```python
from build123d import *

# Parameters (mm, degrees)
BOSS_EXTRUDE1_DEPTH = 0.8
SKETCH2_W           = 9.888461937
SKETCH2_H           = 20
CUT_EXTRUDE1_DEPTH  = 0.8
FILLET1_R           = 1
BOSS_EXTRUDE2_DEPTH = 1
SKETCH4_W           = 5
SKETCH4_H           = 1
BOSS_EXTRUDE3_DEPTH = 1
FILLET2_R           = 1
CUT_EXTRUDE2_DEPTH  = 10


with BuildPart() as part:
    # Sketch1 → Boss-Extrude1 (new body)
    with BuildSketch(Plane(origin=(0, 0, 0), x_dir=(1, 0, 0), z_dir=(0, 1, 0))):
        Polygon((-22, 15), (-23.5, 4.326945416), (-23.5, -4.326945416), (-22, -15), (22, -15), (23.5, -4.326945416), (23.5, 4.326945416), (22, 15), align=None)
    extrude(amount=BOSS_EXTRUDE1_DEPTH)

    # Sketch2 → Cut-Extrude1 (cut)
    with BuildSketch(Plane(origin=(0, 0.8, 0), x_dir=(1, 0, 0), z_dir=(0, 1, 0))):
        with Locations((-21.444230969, 2.5)):
            Rectangle(SKETCH2_W, SKETCH2_H)
    extrude(amount=-CUT_EXTRUDE1_DEPTH, mode=Mode.SUBTRACT)

    # Fillet1
    fillet1_edges = [part.edges().sort_by_distance(p)[0] for p in [
        (-16.5, 0.4, 7.5),
    ]]
    fillet(fillet1_edges, radius=FILLET1_R)

    # Sketch3 → Boss-Extrude2 (add)
    with BuildSketch(Plane.XZ):
        Polygon((-19.5, 13.5), (-20.5, 13.5), (-20.5, 12.5), (-20.5, 8.5), (-19.5, 8.5), (-19.5, 12.5), (-15.5, 12.5), (-15.5, 13.5), align=None)
        Polygon((19.5, 13.5), (15.5, 13.5), (15.5, 12.5), (19.5, 12.5), (19.5, 8.5), (20.5, 8.5), (20.5, 12.5), (20.5, 13.5), align=None)
        Polygon((19.5, -13.5), (20.5, -13.5), (20.5, -12.5), (20.5, -8.5), (19.5, -8.5), (19.5, -12.5), (15.5, -12.5), (15.5, -13.5), align=None)
    extrude(amount=BOSS_EXTRUDE2_DEPTH)

    # Sketch4 → Boss-Extrude3 (add)
    with BuildSketch(Plane.XZ):
        with Locations((-18, -13)):
            Rectangle(SKETCH4_W, SKETCH4_H)
    extrude(amount=BOSS_EXTRUDE3_DEPTH)

    # Fillet2
    fillet2_edges = [part.edges().sort_by_distance(p)[0] for p in [
        (-16.5, 0.4, -12.5),
    ]]
    fillet(fillet2_edges, radius=FILLET2_R)

    # Sketch5 → Cut-Extrude2 (cut)
    with BuildSketch(Plane(origin=(0, 0.8, 0), x_dir=(1, 0, 0), z_dir=(0, 1, 0))):
        Polygon((1.1702653, 5.066019343), (0.081403121, 5.066019343), (2.306192784, 9.380762933), (3.209337816, 9.380762933), (5.432855444, 5.066019343), (4.3452653, 5.066019343), (2.7577653, 8.145616699), align=None)
        Polygon((1.1702653, -6.924365272), (0.081403121, -6.924365272), (2.306192784, -2.609621682), (3.209337816, -2.609621682), (5.432855444, -6.924365272), (4.3452653, -6.924365272), (2.7577653, -3.844767916), align=None)
    extrude(amount=-CUT_EXTRUDE2_DEPTH, mode=Mode.SUBTRACT)


solid = part.part
```
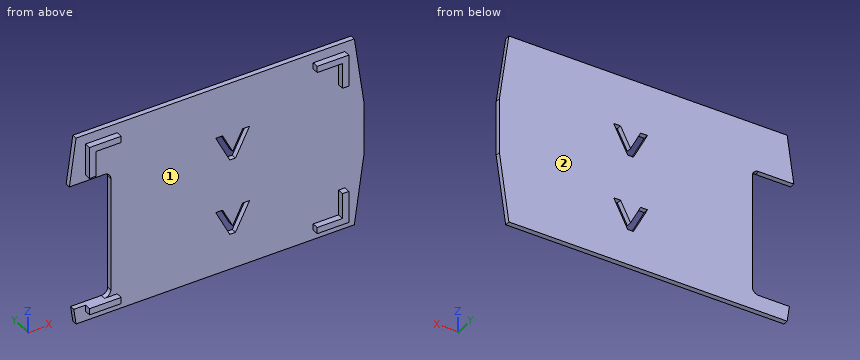
Work out the finished part from the listing and answer in its coordinate system (mm). Face numbers are marked on the shaded views. Round coordinates to 2 decimals unless told otherwise and drop trailing zeros. Loops run counter-clockwise (first coordinate to the right, second up) from the corner with the lowest first, then second, coordinate; pieces in that order, holes last. Notation, with made-up numbers: M 14,76.5 L 66,76.5 A7 ccw 66,89.5 Z; hole C 51.5,78.25 d3. An arc over 180 degrees is marked long. One line per question, with ' | ' between items.
Q1. Find section C-C, the plane x = -2.5. Give the vertices of the cut face in (y, z), then the cut area to 3 significant figures.
Conclusion:
outline: M 0,-15 L 0.8,-15 L 0.8,15 L 0,15 Z | area: 24.0 mm2
Q2. Find section D-D, the plane z = -13. Give the vertices of the cut face in (x, y), then the cut area to 3 significant figures.
Conclusion:
outline: M -22.28,0 L -20.5,0 L -20.5,-1 L -15.5,-1 L -15.5,0 L 15.5,0 L 15.5,-1 L 20.5,-1 L 20.5,0 L 22.28,0 L 22.28,0.8 L -22.28,0.8 Z | area: 45.6 mm2
Q3. Consider line 1 along Z through (x, y) = (16, -0.15); line 2 along X through (y, z) = (-0.4, 9.5); line 3 along X through (y, z) = (0.7, 5). Determine where each line is inside the solid, lowest interval first. Write a range as from..to.
Conclusion:
line 1: z = -13.5..-12.5, 12.5..13.5 | line 2: x = -20.5..-19.5, 19.5..20.5 | line 3: x = -16.5..1.07, 2.16..3.35, 4.44..23.41
Q4. Each of these flat-tipped pins is pushed along its axis until it touches: pin 1 Ø0.9 at (x, y) = (-19.5, -0.5) entering from +Z; pin 2 Ø0.9 at (y, z) = (0.5, 1) entering from -X; pin 3 Ø0.5 at (y, z) = (-0.5, 10) entering from -X. Where does it stop, or does it pass through?
Conclusion:
pin 1: stops at z = 13.5 | pin 2: stops at x = -16.5 | pin 3: stops at x = -20.5
Q5. Find section A-A, the plane y = -0.5. Give the vertices of the cut face in (x, z).
Conclusion:
outline: M -20.5,-13.5 L -15.5,-13.5 L -15.5,-12.5 L -20.5,-12.5 Z; M -20.5,8.5 L -19.5,8.5 L -19.5,12.5 L -15.5,12.5 L -15.5,13.5 L -20.5,13.5 Z; M 15.5,-13.5 L 20.5,-13.5 L 20.5,-8.5 L 19.5,-8.5 L 19.5,-12.5 L 15.5,-12.5 Z; M 15.5,12.5 L 19.5,12.5 L 19.5,8.5 L 20.5,8.5 L 20.5,13.5 L 15.5,13.5 Z
Q6. The mould has two halves that part along X. Classify the marked faces 1 and 2: +X half, -X half, draft (parallel to the pull), parting line (faces both ways), or undercut.
Conclusion:
face 1: undercut | face 2: draft
Q7. Find section B-B, the plane z = -6. Give the vertices of the cut face in (x, y), then the cut area to 3 significant figures.
Conclusion:
outline: M -16.5,0 L 0.56,0 L 0.56,0.8 L -16.5,0.8 Z; M 1.65,0 L 3.86,0 L 3.86,0.8 L 1.65,0.8 Z; M 4.95,0 L 23.26,0 L 23.26,0.8 L 4.95,0.8 Z | area: 30.1 mm2
